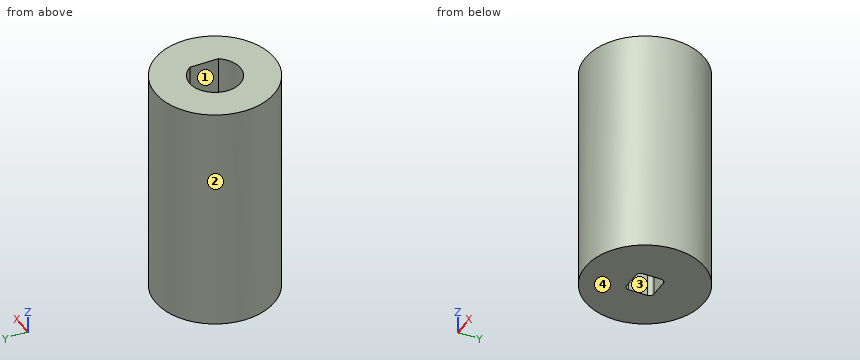
from build123d import *

# Parameters (mm, degrees)
F0_R     = 7
F1_DEPTH = 14.2
F2_R     = 7
F2_R_2   = 5
F3_DEPTH = 3
F4_R     = 7
F4_R_2   = 5
F4_W     = 3.2
F4_H     = 3.2
F5_DEPTH = 10
F6_R     = 0.5


with BuildPart() as f1:
    # F0 (on Top) → F1 (new body)
    with BuildSketch(Plane.XY):
        Circle(F0_R)
        with BuildLine():
            ThreePointArc((2.5, 1.6583123952), (2.8722813233, 0.8660254038), (3, 0))
            ThreePointArc((3, 0), (2.8722813233, -0.8660254038), (2.5, -1.6583123952))
            ThreePointArc((2.5, -1.6583123952), (-0.8660254038, -2.8722813233), (-3, 0))
            ThreePointArc((-3, 0), (-0.8660254038, 2.8722813233), (2.5, 1.6583123952))
        make_face(mode=Mode.SUBTRACT)
        with BuildLine():
            ThreePointArc((2.5, -1.6583123952), (2.8722813233, -0.8660254038), (3, 0))
            ThreePointArc((3, 0), (2.8722813233, 0.8660254038), (2.5, 1.6583123952))
            Line((2.5, 1.6583123952), (2.5, 0))
            Line((2.5, 0), (2.5, -1.6583123952))
        make_face()
    extrude(amount=F1_DEPTH)

    # F2 (on face) → F3 (join)
    with BuildSketch(Plane(origin=(0, 0, 0), x_dir=(1, 0, 0), z_dir=(0, 0, -1))):
        Circle(F2_R)
        Circle(F2_R_2, mode=Mode.SUBTRACT)
        Circle(F2_R_2)
        with BuildLine():
            ThreePointArc((2.5, -1.6583123952), (-3, 0), (2.5, 1.6583123952))
            Line((2.5, 1.6583123952), (2.5, -1.6583123952))
        make_face(mode=Mode.SUBTRACT)
        with BuildLine():
            Line((2.5, -1.6583123952), (2.5, 1.6583123952))
            ThreePointArc((2.5, 1.6583123952), (-3, 0), (2.5, -1.6583123952))
        make_face()
    extrude(amount=F3_DEPTH)

    # F4 (on face) → F5 (join)
    with BuildSketch(Plane(origin=(0, 0, -3), x_dir=(1, 0, 0), z_dir=(0, 0, -1))):
        Circle(F4_R)
        Circle(F4_R_2, mode=Mode.SUBTRACT)
        Circle(F4_R_2)
        Rectangle(F4_W, F4_H, mode=Mode.SUBTRACT)
    extrude(amount=F5_DEPTH)

    # F6
    f6_edges = [f1.edges().sort_by_distance(p)[0] for p in [
        (-1.6, -1.6, -8),
        (-1.6, 1.6, -8),
        (1.6, -1.6, -8),
        (1.6, 1.6, -8),
    ]]
    fillet(f6_edges, radius=F6_R)


solid = f1.part
Can you work these out from the model? Positions are in its coordinate system, mm. Face numbers are marked on the shaded views. Coordinates: 2 decimals unless noted, no trailing zeros. Write each loop counter-clockwise with the first axis right and the second up, starting at its lowest first coordinate (ties: lowest second). Pieces come first, ordered by that corner, then holes. Notation, with made-up numbers: M 88,74 L 146,74 A14 ccw 146,86 Z; hole C -8,1 d4. An arc over 180 degrees is marked long. Use one line per item in the form item = value.
Q1. If we section it at D-D (y = 5.5): Write out the boundary of the cut face in (x, z), then the cut area to 3 significant figures.
Model answer:
outline = M -4.33,-13 L 4.33,-13 L 4.33,14.2 L -4.33,14.2 Z
area = 236 mm^2
Q2. If we section it at B-B (x = 0): Write out the boundary of the cut face in (y, z).
Model answer:
outline = M -7,-13 L -1.6,-13 L -1.6,-3 L 1.6,-3 L 1.6,-13 L 7,-13 L 7,14.2 L 3,14.2 L 3,0 L -3,0 L -3,14.2 L -7,14.2 Z
Q3. We'd pull the mould along X, two halves only. Please class the marked faces 1, 2, 3 and 4: +X half, -X half, draft (parallel to the pull), parting line (faces both ways), or undercut.
Model answer:
face_1 = undercut
face_2 = parting line
face_3 = undercut
face_4 = draft
Q4. If we section it at A-A (z = -5.5): Write out the boundary of the cut face in (x, y), then the cut area to 3 significant figures.
Model answer:
outline = C 0,0 d14; hole M -1.6,-1.1 A0.5 ccw -1.1,-1.6 L 1.1,-1.6 A0.5 ccw 1.6,-1.1 L 1.6,1.1 A0.5 ccw 1.1,1.6 L -1.1,1.6 A0.5 ccw -1.6,1.1 Z
area = 144 mm^2
Q5. If we section it at C-C (z = -0.75): Write out the boundary of the cut face in (x, y), then the cut area to 3 significant figures.
Model answer:
outline = C 0,0 d14
area = 154 mm^2
Q6. For P1, Ø2, axis at x = 3, z = -2, coming from the +Y side; P2, Ø4, axis at y = -3, z = 11, coming from the +X side; P3, Ø8, axis at y = 5.5, z = -5.5, coming from the -X side, each with a flat end and sliding along its axis, tell me the tip position at first contact or that it passes through.
Model answer:
P1 = 6.71
P2 = 6.93
P3 = -6.84
Q7. I need wall thicknesses on line 1 along Y through (x, z) = (0, 3.5); line 2 along Y through (x, z) = (1.75, 5.25); line 3 along X through (y, z) = (-1, 9.25). Which ranges of each line are inside material? Lowest first, please. Write a range as from..to.
Model answer:
line_1 = -7..-3, 3..7
line_2 = -6.78..-2.44, 2.44..6.78
line_3 = -6.93..-2.83, 2.5..6.93
